from build123d import *

# Parameters (mm, degrees)
SKETCH1_R           = 12.7
BOSS_EXTRUDE1_DEPTH = 12.7
SKETCH2_R           = 17.78
BOSS_EXTRUDE2_DEPTH = 3.048
SKETCH9_R           = 6.477
CUT_EXTRUDE5_DEPTH  = 2.286
SKETCH10_R          = 6.731
CUT_EXTRUDE6_DEPTH  = 4.064
SKETCH11_R          = 5.207
CUT_EXTRUDE7_DEPTH  = 29.169962726


with BuildPart() as part:
    # Sketch1 → Boss-Extrude1 (new body)
    with BuildSketch(Plane.XY):
        Circle(SKETCH1_R)
    extrude(amount=BOSS_EXTRUDE1_DEPTH)

    # Sketch2 → Boss-Extrude2 (add, symmetric)
    with BuildSketch(Plane.XY.offset(6.35)):
        with Locations(Location((0, 0, 0), (0, 0, 180))):
            Circle(SKETCH2_R)
    extrude(amount=BOSS_EXTRUDE2_DEPTH, both=True)

    # Sketch9 → Cut-Extrude5 (cut, symmetric)
    with BuildSketch(Plane.XY.offset(6.35)):
        Circle(SKETCH9_R)
    extrude(amount=CUT_EXTRUDE5_DEPTH, both=True, mode=Mode.SUBTRACT)

    # Sketch10 → Cut-Extrude6 (cut)
    with BuildSketch(Plane(origin=(0, 0, 0), x_dir=(-1, 0, 0), z_dir=(0, 0, -1))):
        Circle(SKETCH10_R)
    extrude(amount=-CUT_EXTRUDE6_DEPTH, mode=Mode.SUBTRACT)

    # Sketch11 → Cut-Extrude7 (cut, through all)
    with BuildSketch(Plane.XY.offset(12.7)):
        Circle(SKETCH11_R)
    extrude(amount=-CUT_EXTRUDE7_DEPTH, mode=Mode.SUBTRACT)


solid = part.part
Part model, mm, in its own coordinate system. A direction names the side the tool comes from. Give positions to 0.01 mm unless a question says otherwise; leave off trailing zeros. Order: outer loops, then holes, each group sorted by start corner. A loop starts at its lowest first (then second) coordinate and runs counter-clockwise, first axis right, second up. Notation, with made-up numbers: (-35.5, 10) - (23.5, 10) arc R10 ccw to (23.5, 26) - close; hole circle Ø7 at (58, -26.75). An arc over 180 degrees is marked (long way). Use a Markdown table: item, result.
1) Two-plate mould, pull along X, no slides. Class faces 1 (the flat face through (5, -5, 0)), 2 (the cylindrical face through (-1.404, -6.323, 6.382)), 3 (the cylindrical face through (-2.75, -12.4, 11.03)): +X half, -X half, draft (parallel to the pull), parting line (faces both ways), or undercut.
Checked values:
| item | result |
|---|---|
| face 1 | draft |
| face 2 | undercut |
| face 3 | parting line |
2) Saw through at A-A on x = 0. List the corners of the cut face in (y, z), plus the area to 3 significant figures.
Checked values:
| item | result |
|---|---|
| outline | (-17.78, 3.3) - (-12.7, 3.3) - (-12.7, 0) - (-6.73, 0) - (-6.73, 4.06) - (-6.48, 4.06) - (-6.48, 8.64) - (-5.21, 8.64) - (-5.21, 12.7) - (-12.7, 12.7) - (-12.7, 9.4) - (-17.78, 9.4) - close; (5.21, 8.64) - (6.48, 8.64) - (6.48, 4.06) - (6.73, 4.06) - (6.73, 0) - (12.7, 0) - (12.7, 3.3) - (17.78, 3.3) - (17.78, 9.4) - (12.7, 9.4) - (12.7, 12.7) - (5.21, 12.7) - close |
| area | 228 mm² |
3) Saw through at D-D on y = -12. List the corners of the cut face in (x, z).
Checked values:
| item | result |
|---|---|
| outline | (-13.12, 3.3) - (-4.16, 3.3) - (-4.16, 0) - (4.16, 0) - (4.16, 3.3) - (13.12, 3.3) - (13.12, 9.4) - (4.16, 9.4) - (4.16, 12.7) - (-4.16, 12.7) - (-4.16, 9.4) - (-13.12, 9.4) - close |
4) 3-axis set-ups, long thin cutter, end or side, ignore diameter. For faces 4 (the flat face through (-12, 8, 9.398)), 5 (the flat face through (5.5, 0.2, 12.7)), 6 (the cylindrical face through (-2.75, -12.4, 1.63)): which of +Z, -Z, +X, -X, +Y, -Y reach the whole face in a straight line?
Checked values:
| item | result |
|---|---|
| face 4 | +Z |
| face 5 | +Z, +X, -X, +Y, -Y |
| face 6 | -Z |
5) Saw through at C-C on z = 6.5. List the corners of the cut face in (x, y).
Checked values:
| item | result |
|---|---|
| outline | circle Ø35.56 at (0, 0); hole circle Ø12.95 at (0, 0) |
6) Probe L1, parallel to Z at x = 9, y = 10; L2, parallel to Y at x = 0, z = 7.45; L3, parallel to Y at x = 5, z = 1. List the from-to ranges inside material, lowest first. Write a range as from..to.
Checked values:
| item | result |
|---|---|
| L1 | 3.3..9.4 |
| L2 | -17.78..-6.48, 6.48..17.78 |
| L3 | -11.67..-4.51, 4.51..11.67 |
7) Flat gauge pins, fed straight in: P1, Ø12, axis at x = 0, y = 0, coming from the +Z side; P2, Ø3, axis at y = -5, z = 11, coming from the -X side; P3, Ø1.5, axis at x = 8.5, y = 12.5, coming from the +Z side; P4, Ø2, axis at y = -11, z = 3, coming from the +X side. Where does each tip first touch, or does it go through?
Checked values:
| item | result |
|---|---|
| P1 | z = 12.7 |
| P2 | x = -12.21 |
| P3 | z = 9.4 |
| P4 | x = 14.67 |
